from build123d import *

# Parameters (mm, degrees)
BASE_FLANGE1_DEPTH               = 2.5908
EDGE_FLANGE1_STRIP_W             = 15.4432
EDGE_FLANGE1_STRIP_H             = 2.5908
EDGE_FLANGE1_STRIP_CUT_DEPTH     = 1219.2
EDGE_FLANGE1_DEPTH               = 1219.2
F_17_64_0_26563_DIAMETER_HOLE1_D = 6.747002
FILLET1_R                        = 3.175
F_17_64_0_26563_DIAMETER_HOLE2_D = 6.747002
F_17_64_0_26563_DIAMETER_HOLE3_D = 6.747002


# Sheet-metal steps are written as plain solids
with BuildPart() as part:
    # Sketch2 → Base-Flange1 (new body)
    with BuildSketch(Plane(origin=(0, 0, 0), x_dir=(1, 0, 0), z_dir=(0, 1, 0))):
        Polygon((0, 0), (1219.2, 0), (1219.2, 50.8), (-19.05, 50.8), (-19.05, 19.05), (0, 9.525), align=None)
    extrude(amount=-BASE_FLANGE1_DEPTH)

    # Edge-Flange1 strip (across the edge) → Edge-Flange1 strip cut (cut)
    with BuildSketch(Plane(origin=(0, 0, 0), x_dir=(0, 0, -1), z_dir=(1, 0, 0))):
        with Locations((-2.5908, -1.2954)):
            Rectangle(EDGE_FLANGE1_STRIP_W, EDGE_FLANGE1_STRIP_H)
    extrude(amount=EDGE_FLANGE1_STRIP_CUT_DEPTH, mode=Mode.SUBTRACT)

    # Edge-Flange1 section (across the edge) → Edge-Flange1 (add)
    with BuildSketch(Plane(origin=(0, 0, 0), x_dir=(0, 0, -1), z_dir=(1, 0, 0))):
        with BuildLine():
            Line((0, 2.54), (0, 48.2092))
            Line((0, 48.2092), (2.5908, 48.2092))
            Line((2.5908, 48.2092), (2.5908, 2.54))
            ThreePointArc((2.5908, 2.54), (3.334748776, 0.743948776), (5.1308, 0))
            Line((5.1308, 0), (5.1308, -2.5908))
            ThreePointArc((5.1308, -2.5908), (1.502776527, -1.088023473), (0, 2.54))
        make_face()
    extrude(amount=EDGE_FLANGE1_DEPTH)

    # 17/64 (0.26563) Diameter Hole1 (through all)
    with Locations(Plane(origin=(0, 0, 0), x_dir=(1, 0, 0), z_dir=(0, 1, 0))):
        with Locations((1193.8, 27.305)):
            Hole(F_17_64_0_26563_DIAMETER_HOLE1_D / 2)

    # Fillet1
    fillet1_edges = [part.edges().sort_by_distance(p)[0] for p in [
        (0, -1.2954, -9.525),
        (-19.05, -1.2954, -19.05),
        (-19.05, -1.2954, -50.8),
        (1219.2, -1.2954, -50.8),
        (0, 48.2092, -1.2954),
        (1219.2, 48.2092, -1.2954),
    ]]
    fillet(fillet1_edges, radius=FILLET1_R)

    # 17/64 (0.26563) Diameter Hole2 (through all)
    with Locations(Plane(origin=(0, 0, 0), x_dir=(1, 0, 0), z_dir=(0, 1, 0))):
        with Locations((3.81, 33.3375)):
            Hole(F_17_64_0_26563_DIAMETER_HOLE2_D / 2)

    # 17/64 (0.26563) Diameter Hole3 (through all)
    with Locations(Plane(origin=(0, -2.5908, 0), x_dir=(-1, 0, 0), z_dir=(0, -1, 0))):
        with Locations((-103.6574, 33.655), (-1102.8934, 33.655)):
            Hole(F_17_64_0_26563_DIAMETER_HOLE3_D / 2)


solid = part.part
Here's how the part is built. I have some questions about the finished solid (model axes, mm). A direction names the side the tool comes from. Coordinates: 2 decimals unless noted, no trailing zeros. Order: outer loops, then holes, each group sorted by start corner. A loop starts at its lowest first (then second) coordinate and runs counter-clockwise, first axis right, second up. Notation, with made-up numbers: (21.25, -28.5) -> (42.25, -28.5) arc R35 cw to (42.25, 9.5) -> close; hole circle Ø9 at (53, 73.25). An arc over 180 degrees is marked (long way). Answer in a Markdown table with one row per item.
(1) On a 3-axis mill with a long thin cutter (end or side, diameter ignored), from which of +Z, -Z, +X, -X, +Y, -Y can I reach the whole of each face in a straight line? I mean faces 1 (the face through (1219.2, -2, -13)), 2 (the face through (591, 0, -28)). Say none if no direction works.
Answer key:
| item | result |
|---|---|
| face 1 | +Z, -Z, +X, +Y, -Y |
| face 2 | -Z, +X, -X, +Y |
(2) Will these pins go through, and if not, where does the flat tip stop? pin 1 Ø8 at (x, y) = (528.5, 29.5) entering from -Z; pin 2 Ø23 at (x, z) = (834, -28) entering from +Y; pin 3 Ø6 at (y, z) = (28.5, -5.5) entering from -X.
Answer key:
| item | result |
|---|---|
| pin 1 | z = -2.59 |
| pin 2 | y = 0 |
| pin 3 | x = 0 |
(3) I want a section at B-B on y = 33.5. List the corners of the cut face in (x, z) for me, then the cut area to 3 significant figures.
Answer key:
| item | result |
|---|---|
| outline | (0, -2.59) -> (1219.2, -2.59) -> (1219.2, 0) -> (0, 0) -> close |
| area | 3,160 mm^2 |
(4) I want a section at A-A on x = 352. List the corners of the cut face in (y, z) for me, then the cut area to 3 significant figures.
Answer key:
| item | result |
|---|---|
| outline | (-2.59, -50.8) -> (0, -50.8) -> (0, -5.13) arc R2.54 cw to (2.54, -2.59) -> (48.21, -2.59) -> (48.21, 0) -> (2.54, 0) arc R5.13 ccw to (-2.59, -5.13) -> close |
| area | 252 mm^2 |
(5) Please list where these lines run through material, in increasing order: probe 1 along Z at (x, y) = (3.81, -1.5); probe 2 along Z at (x, y) = (645, 19.5).
Answer key:
| item | result |
|---|---|
| probe 1 | -50.8 to -36.71, -29.96 to -1.97 |
| probe 2 | -2.59 to 0 |
